Could you check a few things on this model? Use its own coordinates, in mm. Face numbers are marked on the shaded views. A direction names the side the tool comes from. Coordinates: 2 decimals unless noted, no trailing zeros. Write each loop counter-clockwise with the first axis right and the second up, starting at its lowest first coordinate (ties: lowest second). Pieces come first, ordered by that corner, then holes. Notation, with made-up numbers: (43, 69) - (52, 69) arc R15 ccw to (52, 78) - close; hole circle Ø6 at (-25.75, 70.5). An arc over 180 degrees is marked (long way). Answer as a JSON object with one key per item and string values. Group by question number.
1) We'd pull the mould along X, two halves only. Please class the marked faces 6, 7, 8 and 9: released by +X, released by -X, zero draft, split by the parting line, or undercut.
2) Will these pins go through, and if not, where does the flat tip stop? pin 1 Ø1.5 at (y, z) = (0, 1) entering from -X; pin 2 Ø1.5 at (x, y) = (-3, 1.5) entering from +Z (3 decimals); pin 3 Ø1.5 at (x, z) = (-5, -0.5) entering from -Y.
3) If we section it at C-C (x = 0.25): Write out the boundary of the cut face in (y, z), plus the area to 3 significant figures.
4) Please list where these lines run through material, in increasing order: line 1 along X through (y, z) = (1.5, 0); line 2 along X through (y, z) = (0.6, 0.8); line 3 along Z through (x, y) = (-4, 0.45).
5) On a 3-axis mill with a long thin cutter (end or side, diameter ignored), from which of +Z, -Z, +X, -X, +Y, -Y can I reach the whole of each face in a straight line? I mean the marked faces 1, 2, 3, 4 and 5. Say none if no direction works.
6) If we section it at B-B (z = 0): Write out the boundary of the cut face in (x, y) (3 decimals), plus the area to 3 significant figures.
7) If we section it at A-A (y = 0.25): Write out the boundary of the cut face in (x, z) (3 decimals).
8) If we section it at D-D (x = -3.5): Write out the boundary of the cut face in (y, z).
```python
from build123d import *

# Parameters (mm, degrees)
BOSS_EXTRUDE1_DEPTH = 2.5
SKETCH4_R           = 0.35
THROUGH_HOLES_DEPTH = 7.493265742
FILLET1_R           = 0.125
SKETCH5_R           = 0.125
BOSS_EXTRUDE2_DEPTH = 0.5


with BuildPart() as part:
    # Sketch3 → Boss-Extrude1 (new body)
    with BuildSketch(Plane(origin=(0, 0, 0), x_dir=(1, 0, 0), z_dir=(0, 1, 0))):
        with BuildLine():
            Line((-2.5, 0.9), (-2, 0.93))
            Line((-2, 0.93), (-2, 0.56))
            Line((-2, 0.56), (-1.5, 0.56))
            Line((-1.5, 0.56), (-1.5, 0.96))
            Line((-1.5, 0.96), (0, 1.05))
            ThreePointArc((0, 1.05), (1.05, 0), (0, -1.05))
            Line((0, -1.05), (-1.5, -0.96))
            Line((-1.5, -0.96), (-1.5, -0.56))
            Line((-1.5, -0.56), (-2, -0.56))
            Line((-2, -0.56), (-2, -0.93))
            Line((-2, -0.93), (-2.5, -0.9))
            Line((-2.5, -0.9), (-5, -0.9))
            ThreePointArc((-5, -0.9), (-5.9, 0), (-5, 0.9))
            Line((-5, 0.9), (-2.5, 0.9))
        make_face()
    extrude(amount=BOSS_EXTRUDE1_DEPTH)

    # Sketch4 → Through Holes (cut, through all)
    with BuildSketch(Plane(origin=(0, 2.5, 0), x_dir=(1, 0, 0), z_dir=(0, 1, 0))):
        with Locations(Location((0, 0, 0), (0, 0, 270))):
            Circle(SKETCH4_R)
        with BuildLine():
            Line((-4.79, -0.9), (-4.37, -0.9))
            Line((-4.37, -0.9), (-4.37, 0.21))
            Line((-4.37, 0.21), (-5, 0.21))
            ThreePointArc((-5, 0.21), (-5.21, 0), (-5, -0.21))
            Line((-5, -0.21), (-4.79, -0.21))
            Line((-4.79, -0.21), (-4.79, -0.9))
        make_face()
    extrude(amount=-THROUGH_HOLES_DEPTH, mode=Mode.SUBTRACT)

    # Fillet1
    fillet1_edges = [part.edges().sort_by_distance(p)[0] for p in [
        (-2, 1.25, 0.56),
        (-1.5, 1.25, 0.56),
        (-1.5, 1.25, -0.56),
        (-2, 1.25, -0.56),
        (-4.37, 1.25, 0.9),
        (-4.79, 1.25, 0.9),
    ]]
    fillet(fillet1_edges, radius=FILLET1_R)

    # Sketch5 → Boss-Extrude2 (add)
    with BuildSketch(Plane(origin=(0, 0, 0), x_dir=(1, 0, 0), z_dir=(0, 1, 0))):
        with BuildLine():
            Line((-1.514973073, -1.209551211), (-1.514973073, 1.209551211))
            Line((-1.514973073, 1.209551211), (-0.007892579, 1.299976041))
            ThreePointArc((-0.007892579, 1.299976041), (1.3, 0), (-0.007892579, -1.299976041))
            Line((-0.007892579, -1.299976041), (-1.514973073, -1.209551211))
        make_face()
        with Locations(Location((0, 0, 0), (0, 0, 270))):
            Circle(SKETCH5_R, mode=Mode.SUBTRACT)
    extrude(amount=-BOSS_EXTRUDE2_DEPTH)


solid = part.part
```
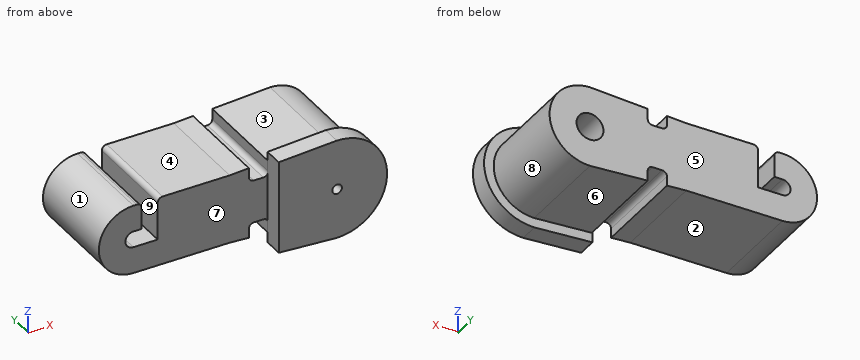
Here are the results:
{
 "1": {"face 6": "released by -X", "face 7": "zero draft", "face 8": "released by +X", "face 9": "undercut"},
 "2": {"pin 1": "stops at x = -5.86", "pin 2": "stops at z = 0.915", "pin 3": "stops at y = 0"},
 "3": {"outline": "(-0.5, -1.28) - (0, -1.28) - (0, -1.02) - (2.5, -1.02) - (2.5, -0.24) - (0, -0.24) - (0, 0.24) - (2.5, 0.24) - (2.5, 1.02) - (0, 1.02) - (0, 1.28) - (-0.5, 1.28) - close", "area": "5.15 mm²"},
 "4": {"line 1": "x = -5.9 to -5.21, -4.37 to -0.35, 0.35 to 1.05", "line 2": "x = -5.41 to -4.79, -4.37 to -2, -1.5 to 0.68", "line 3": "z = -0.9 to 0.9"},
 "5": {"face 1": "-X, +Y, -Y", "face 2": "-Z, -X, +Y, -Y", "face 3": "+Z, -X, +Y", "face 4": "+Z, -X, +Y, -Y", "face 5": "+Z, -Z, +X, -X, +Y"},
 "6": {"outline": "(-5.9, 0) - (-5.21, 0) - (-5.21, 2.5) - (-5.9, 2.5) - close; (-4.37, 0) - (-1.515, 0) - (-1.515, -0.5) - (-0.125, -0.5) - (-0.125, 0) - (-0.35, 0) - (-0.35, 2.5) - (-4.37, 2.5) - close; (0.125, -0.5) - (1.3, -0.5) - (1.3, 0) - (1.05, 0) - (1.05, 2.5) - (0.35, 2.5) - (0.35, 0) - (0.125, 0) - close", "area": "14.8 mm²"},
 "7": {"outline": "(-5, -0.9) - (-2.5, -0.9) - (-2, -0.93) - (-2, -0.685) arc R0.125 cw to (-1.875, -0.56) - (-1.625, -0.56) arc R0.125 cw to (-1.5, -0.685) - (-1.5, -0.96) - (0, -1.05) arc R1.05 ccw to (0, 1.05) - (-1.5, 0.96) - (-1.5, 0.685) arc R0.125 cw to (-1.625, 0.56) - (-1.875, 0.56) arc R0.125 cw to (-2, 0.685) - (-2, 0.93) - (-2.5, 0.9) - (-4.245, 0.9) arc R0.125 ccw to (-4.37, 0.775) - (-4.37, -0.21) - (-5, -0.21) arc R0.21 cw to (-5, 0.21) - (-4.79, 0.21) - (-4.79, 0.775) arc R0.125 ccw to (-4.915, 0.9) - (-5, 0.9) arc R0.9 ccw to start; hole circle Ø0.7 at (0, 0)"},
 "8": {"outline": "(0, -0.9) - (2.5, -0.9) - (2.5, 0.9) - (0, 0.9) - close"}
}
